from build123d import *

# Parameters (mm, degrees)
BOSS_EXTRUDE1_DEPTH = 7
SKETCH2_R           = 2.75
BOSS_EXTRUDE2_DEPTH = 2.1
SKETCH3_R           = 1.5
BOSS_EXTRUDE3_DEPTH = 8.5
SKETCH4_R           = 1.5
CUT_EXTRUDE1_DEPTH  = 5
SKETCH5_R           = 0.8
CUT_EXTRUDE2_DEPTH  = 14.378714437


with BuildPart() as part:
    # Sketch1 → Boss-Extrude1 (new body)
    with BuildSketch(Plane.YZ):
        Polygon((3.4, 0), (1.7, 2.944486373), (-1.7, 2.944486373), (-3.4, 0), (-1.7, -2.944486373), (1.7, -2.944486373), align=None)
    extrude(amount=BOSS_EXTRUDE1_DEPTH)

    # Sketch2 → Boss-Extrude2 (add)
    with BuildSketch(Plane.YZ.offset(7)):
        with Locations(Location((0, 0, 0), (0, 0, 270))):
            Circle(SKETCH2_R)
    extrude(amount=BOSS_EXTRUDE2_DEPTH)

    # Sketch3 → Boss-Extrude3 (add)
    with BuildSketch(Plane.YZ.offset(9.1)):
        with Locations(Location((0, 0, 0), (0, 0, 270))):
            Circle(SKETCH3_R)
    extrude(amount=BOSS_EXTRUDE3_DEPTH)

    # Sketch4 → Cut-Extrude1 (cut)
    with BuildSketch(Plane(origin=(0, 0, 0), x_dir=(0, -1, 0), z_dir=(-1, 0, 0))):
        with Locations(Location((0, 0, 0), (0, 0, 270))):
            Circle(SKETCH4_R)
    extrude(amount=-CUT_EXTRUDE1_DEPTH, mode=Mode.SUBTRACT)

    # Sketch5 → Cut-Extrude2 (cut, through all)
    with BuildSketch(Plane(origin=(5, 0, 0), x_dir=(0, -1, 0), z_dir=(-1, 0, 0))):
        with Locations(Location((0, 0, 0), (0, 0, 90))):
            Circle(SKETCH5_R)
    extrude(amount=-CUT_EXTRUDE2_DEPTH, mode=Mode.SUBTRACT)


solid = part.part
For this review, take the finished solid that the model builds, in its own axes (mm). A direction names the side the tool comes from. Coordinates: 2 decimals unless noted, no trailing zeros. Order: outer loops, then holes, each group sorted by start corner. A loop starts at its lowest first (then second) coordinate and runs counter-clockwise, first axis right, second up. Notation, with made-up numbers: (-7, 8.5) - (3, 8.5) arc R16 ccw to (3, 25.5) - close; hole circle Ø7 at (42, 71.5). An arc over 180 degrees is marked (long way). Answer as CSV lines item,"result". Start each with the question number.
1) Insertion check: P1, Ø3, axis at x = 15, z = 1, coming from the +Y side. The pin has a flat end and moves straight along its axis. Give the tip position at first contact, or say it passes through.
2) Add section D-D (y = -2.5). State the section outline as (x, z) points, then the cut area to 3 significant figures.
3) Add section A-A (y = 0). State the section outline as (x, z) points, then the cut area to 3 significant figures.
4) Add section B-B (x = 3.5). State the section outline as (y, z) points, then the cut area to 3 significant figures.
5) Draft analysis for pull direction Y (two halves, no side actions). For faces 4 (the cylindrical face through (2.46, -0.45, -1.43)), 5 (the flat face through (3.45, -2.54, 1.49)), 6 (the cylindrical face through (13.29, 0.45, -1.43)), state which applies: +Y half, -Y half, draft (parallel to the pull), parting line (faces both ways), or undercut.
6) Machinability: for faces 1 (the cylindrical face through (11.21, -0.49, -0.63)), 2 (the cylindrical face through (8.035, -2.685, 0.596)), 3 (the flat face through (5, 1, 0)), which of the approach directions +Z, -Z, +X, -X, +Y, -Y give a long, thin tool a straight path to every point of the face, cutting with its end or side? Answer none if there is none.
7) To check wall thickness, follow line 1 along Y through (x, z) = (13.75, 0); line 2 along Y through (x, z) = (2.25, 0.3); line 3 along X through (y, z) = (-2, -0.3). State the ranges of each line that lie inside material, in increasing order. Write a range as [from, to].
8) Add section C-C (z = -0.5). State the section outline as (x, y) points, then the cut area to 3 significant figures.
Result:
1,P1,"y = 1.5"
2,outline,"(0, -1.56) - (7, -1.56) - (7, -1.15) - (9.1, -1.15) - (9.1, 1.15) - (7, 1.15) - (7, 1.56) - (0, 1.56) - close"
2,area,"26.6 mm^2"
3,outline,"(0, -2.94) - (7, -2.94) - (7, -2.75) - (9.1, -2.75) - (9.1, -1.5) - (17.6, -1.5) - (17.6, -0.8) - (5, -0.8) - (5, -1.5) - (0, -1.5) - close; (0, 1.5) - (5, 1.5) - (5, 0.8) - (17.6, 0.8) - (17.6, 1.5) - (9.1, 1.5) - (9.1, 2.75) - (7, 2.75) - (7, 2.94) - (0, 2.94) - close"
3,area,"43.1 mm^2"
4,outline,"(-3.4, 0) - (-1.7, -2.94) - (1.7, -2.94) - (3.4, 0) - (1.7, 2.94) - (-1.7, 2.94) - close; hole circle Ø3 at (0, 0)"
4,area,"23.0 mm^2"
5,face 4,"undercut"
5,face 5,"-Y half"
5,face 6,"parting line"
6,face 1,"+X, -X"
6,face 2,"+X"
6,face 3,"-X"
7,line 1,"[-1.5, -0.8], [0.8, 1.5]"
7,line 2,"[-3.23, -1.47], [1.47, 3.23]"
7,line 3,"[0, 9.1]"
8,outline,"(0, -3.11) - (7, -3.11) - (7, -2.7) - (9.1, -2.7) - (9.1, -1.41) - (17.6, -1.41) - (17.6, -0.62) - (5, -0.62) - (5, -1.41) - (0, -1.41) - close; (0, 1.41) - (5, 1.41) - (5, 0.62) - (17.6, 0.62) - (17.6, 1.41) - (9.1, 1.41) - (9.1, 2.7) - (7, 2.7) - (7, 3.11) - (0, 3.11) - close"
8,area,"49.1 mm^2"
